Part model, mm, in its own coordinate system. A direction names the side the tool comes from. Round coordinates to 2 decimals unless told otherwise and drop trailing zeros. Write each loop counter-clockwise with the first axis right and the second up, starting at its lowest first coordinate (ties: lowest second). Pieces come first, ordered by that corner, then holes.
```python
from build123d import *

# Parameters (mm, degrees)
SKETCH1_W            = 15.8
SKETCH1_H            = 3.2
BOSS_EXTRUDE1_DEPTH  = 7.8
SKETCH2_R            = 2.4
BOSS_EXTRUDE2_DEPTH  = 1.6
LPATTERN1_COUNT      = 2
LPATTERN1_PITCH      = 8
LPATTERN1_COUNT_DIR2 = 6
LPATTERN1_PITCH_DIR2 = 8
SHELL1_T             = -1.2
SKETCH3_R            = 1.5
SKETCH3_R_2          = 0.6
BOSS_EXTRUDE3_DEPTH  = 1.8


with BuildPart() as part:
    # Sketch1 → Boss-Extrude1 (new body)
    with BuildSketch(Plane.XY):
        with Locations((7.9, 1.6)):
            Rectangle(SKETCH1_W, SKETCH1_H)
    extrude(amount=-BOSS_EXTRUDE1_DEPTH)

    # Sketch2 → Boss-Extrude2 (add)
    with BuildSketch(Plane(origin=(0, 3.2, 0), x_dir=(1, 0, 0), z_dir=(0, 1, 0))):
        with Locations(Location((3.9, 3.9, 0), (0, 0, 270))):
            Circle(SKETCH2_R)
    boss_extrude2 = extrude(amount=BOSS_EXTRUDE2_DEPTH)

    # LPattern1: Boss-Extrude2 2 × 6, 10 skipped
    with Locations(*[(j * LPATTERN1_PITCH_DIR2, 0, i * LPATTERN1_PITCH) for i in range(LPATTERN1_COUNT) for j in range(LPATTERN1_COUNT_DIR2) if (i, j) not in ((0, 0), (0, 2), (0, 3), (0, 4), (0, 5), (1, 0), (1, 1), (1, 2), (1, 3), (1, 4), (1, 5))]):
        add(boss_extrude2)

    # Shell1
    shell1_openings = [part.faces().sort_by_distance(p)[0] for p in [
        (7.9, 0, -3.9),
    ]]
    offset(amount=SHELL1_T, openings=shell1_openings, kind=Kind.INTERSECTION)

    # Sketch3 → Boss-Extrude3 (add)
    with BuildSketch(Plane.XZ.offset(-2)):
        with Locations(Location((7.9, -3.9, 0), (0, 0, 90))):
            Circle(SKETCH3_R)
        with Locations(Location((7.9, -3.9, 0), (0, 0, 270))):
            Circle(SKETCH3_R_2, mode=Mode.SUBTRACT)
    extrude(amount=BOSS_EXTRUDE3_DEPTH)


solid = part.part
```
Q1. Cut at C-C on y = 2.5. Write the cut outline in (x, z), plus the area to 3 significant figures.
Values follow:
outline: (0, -7.8) - (15.8, -7.8) - (15.8, 0) - (0, 0) - close; hole circle Ø2.4 at (3.9, -3.9); hole circle Ø2.4 at (11.9, -3.9)
area: 114 mm2
Q2. Cut at A-A on y = 1. Write the cut outline in (x, z), plus the area to 3 significant figures.
Values follow:
outline: (0, -7.8) - (15.8, -7.8) - (15.8, 0) - (0, 0) - close; circle Ø3 at (7.9, -3.9); hole (1.2, -6.6) - (14.6, -6.6) - (14.6, -1.2) - (1.2, -1.2) - close; hole circle Ø1.2 at (7.9, -3.9)
area: 56.8 mm2
Q3. Cut at D-D on z = -0.5. Write the cut outline in (x, y).
Values follow:
outline: (0, 0) - (15.8, 0) - (15.8, 3.2) - (0, 3.2) - close
Q4. Cut at B-B on x = 7.9. Write the cut outline in (y, z), plus the area to 3 significant figures.
Values follow:
outline: (0, -7.8) - (3.2, -7.8) - (3.2, 0) - (0, 0) - (0, -1.2) - (2, -1.2) - (2, -2.4) - (0.2, -2.4) - (0.2, -3.3) - (2, -3.3) - (2, -4.5) - (0.2, -4.5) - (0.2, -5.4) - (2, -5.4) - (2, -6.6) - (0, -6.6) - close
area: 17.4 mm2
Q5. Mould opens along Z. For faces 1 (the flat face through (4, 4.8, -4)), 2 (the cylindrical face through (13.924, 3.989, -2.61)), 3 (the flat face through (1.2, 1, -4)), 4 (the flat face through (8, 2, -7.8)) say: +Z half, -Z half, draft (parallel to the pull), parting line (faces both ways), or undercut.
Values follow:
face 1: draft
face 2: parting line
face 3: undercut
face 4: -Z half
Q6. Drop flat-ended pins along their axis: pin 1 (2.5 mm diameter, centred on x = 7.5, z = -4, fed in from -Y); pin 2 (1.2 mm diameter, centred on x = 3.5, z = -4, fed in from -Y); pin 3 (1 mm diameter, centred on x = 14, z = -3, fed in from -Y). Give the stop position or say it passes through.
Values follow:
pin 1: stops at y = 0.2
pin 2: stops at y = 3.6
pin 3: stops at y = 2
Q7. Which spindle directions (+Z, -Z, +X, -X, +Y, -Y) get a long thin tool onto all of the face, cutting with end or side? Do faces 5 (the flat face through (0, 2, -4)), 6 (the cylindrical face through (8.08, 1.113, -4.472)), 7 (the cylindrical face through (1.77, 3.99, -2.79)). Say none if no direction does.
Values follow:
face 5: +Z, -Z, -X, +Y, -Y
face 6: -Y
face 7: +Y
Q8. Wall check: L1, parallel to X at y = 1.65, z = -3.9; L2, parallel to X at y = 2.85, z = -3.9; L3, parallel to Z at x = 13.25, y = 0.5. Give the ranges that are in metal, low to high.
Values follow:
L1: x = 0 to 1.2, 6.4 to 7.3, 8.5 to 9.4, 14.6 to 15.8
L2: x = 0 to 2.7, 5.1 to 10.7, 13.1 to 15.8
L3: z = -7.8 to -6.6, -1.2 to 0
